The model under review builds one solid part; all positions refer to its coordinate system, in mm. A direction names the side the tool comes from. Round coordinates to 2 decimals unless told otherwise and drop trailing zeros. Write each loop counter-clockwise with the first axis right and the second up, starting at its lowest first coordinate (ties: lowest second). Pieces come first, ordered by that corner, then holes. Notation, with made-up numbers: (88.25, -37) -> (105.25, -37) arc R26 ccw to (105.25, -16) -> close; hole circle Ø3 at (54, 59). An arc over 180 degrees is marked (long way). Use CSV: the item, a comma, the result in double quotes. Start each with the question number.
1) Take a section at A-A, the plane z = 15.87. Give the boundary of the cut face in (x, y) (3 decimals).
2) For pin 1 Ø12 at (y, z) = (6, 67.5) entering from +X (3 decimals); pin 2 Ø2 at (x, y) = (32, 3.5) entering from +Z; pin 3 Ø2 at (x, z) = (-3.5, 59.5) entering from -Y; pin 4 Ø10 at (y, z) = (-13.5, 51) entering from -X, all flat-tipped, find the tip position at first contact; note any pin that passes through.
3) Take a section at C-C, the plane y = 15.5. Give the boundary of the cut face in (x, z) (3 decimals), then the cut area to 3 significant figures.
4) Take a section at B-B, the plane x = -23.5. Give the boundary of the cut face in (y, z), then the cut area to 3 significant figures.
5) Take a section at D-D, the plane z = 85. Give the boundary of the cut face in (x, y) (3 decimals).
6) Wall thickness on probe 1 along Z at (x, y) = (-2, -17); probe 2 along X at (y, z) = (11.5, 7.5) (3 decimals); probe 3 along Z at (x, y) = (59.5, 2): over which ranges is each line inside the solid? List them lowest first. Write a range as [from, to].
7) Machinability: for faces 1 (the face through (58.74, 2.68, 6.33)), 2 (the face through (79.015, 0, 16)), 3 (the face through (7.476, 1.877, 59.58)), which of the approach directions +Z, -Z, +X, -X, +Y, -Y give a long, thin tool a straight path to every point of the face, cutting with its end or side? Answer none if there is none.
from build123d import *

# Parameters (mm, degrees)
SKETCH1_W           = 78.03
SKETCH1_H           = 50
BOSS_EXTRUDE2_DEPTH = 30
SKETCH2_R           = 10
BOSS_EXTRUDE3_DEPTH = 40
SKETCH3_R           = 6.25
BOSS_EXTRUDE8_DEPTH = 63
CHAMFER6_SIZE       = 3


with BuildPart() as part:
    # Sketch1 → Boss-Extrude2 (new body)
    with BuildSketch(Plane.XY):
        Rectangle(SKETCH1_W, SKETCH1_H)
    extrude(amount=BOSS_EXTRUDE2_DEPTH)

    # Sketch2 → Boss-Extrude3 (add)
    with BuildSketch(Plane(origin=(39.015, 0, 0), x_dir=(0, 0, -1), z_dir=(1, 0, 0))):
        with Locations((-15.87, -0.32)):
            Circle(SKETCH2_R)
    extrude(amount=BOSS_EXTRUDE3_DEPTH)

    # Sketch3 → Boss-Extrude8 (add)
    with BuildSketch(Plane.XY.offset(30)):
        with Locations((1.515, 0)):
            Circle(SKETCH3_R)
    extrude(amount=BOSS_EXTRUDE8_DEPTH)

    # Chamfer6
    chamfer6_edges = [part.edges().sort_by_distance(p)[0] for p in [
        (-4.735, 0, 93),
    ]]
    chamfer(chamfer6_edges, length=CHAMFER6_SIZE)


solid = part.part
Values found:
1,outline,"(-39.015, -25) -> (39.015, -25) -> (39.015, -10.32) -> (79.015, -10.32) -> (79.015, 9.68) -> (39.015, 9.68) -> (39.015, 25) -> (-39.015, 25) -> close"
2,pin 1,"x = 7.765"
2,pin 2,"z = 30"
2,pin 3,"y = -4.79"
2,pin 4,"through"
3,outline,"(-39.015, 0) -> (39.015, 0) -> (39.015, 30) -> (-39.015, 30) -> close"
3,area,"2,340 mm²"
4,outline,"(-25, 0) -> (25, 0) -> (25, 30) -> (-25, 30) -> close"
4,area,"1,500 mm²"
5,outline,"circle Ø12.5 at (1.515, 0)"
6,probe 1,"[0, 30]"
6,probe 2,"[-39.015, 39.015]"
6,probe 3,"[6.14, 25.6]"
7,face 1,"+X"
7,face 2,"+Z, -Z, +X, +Y, -Y"
7,face 3,"+Z"
